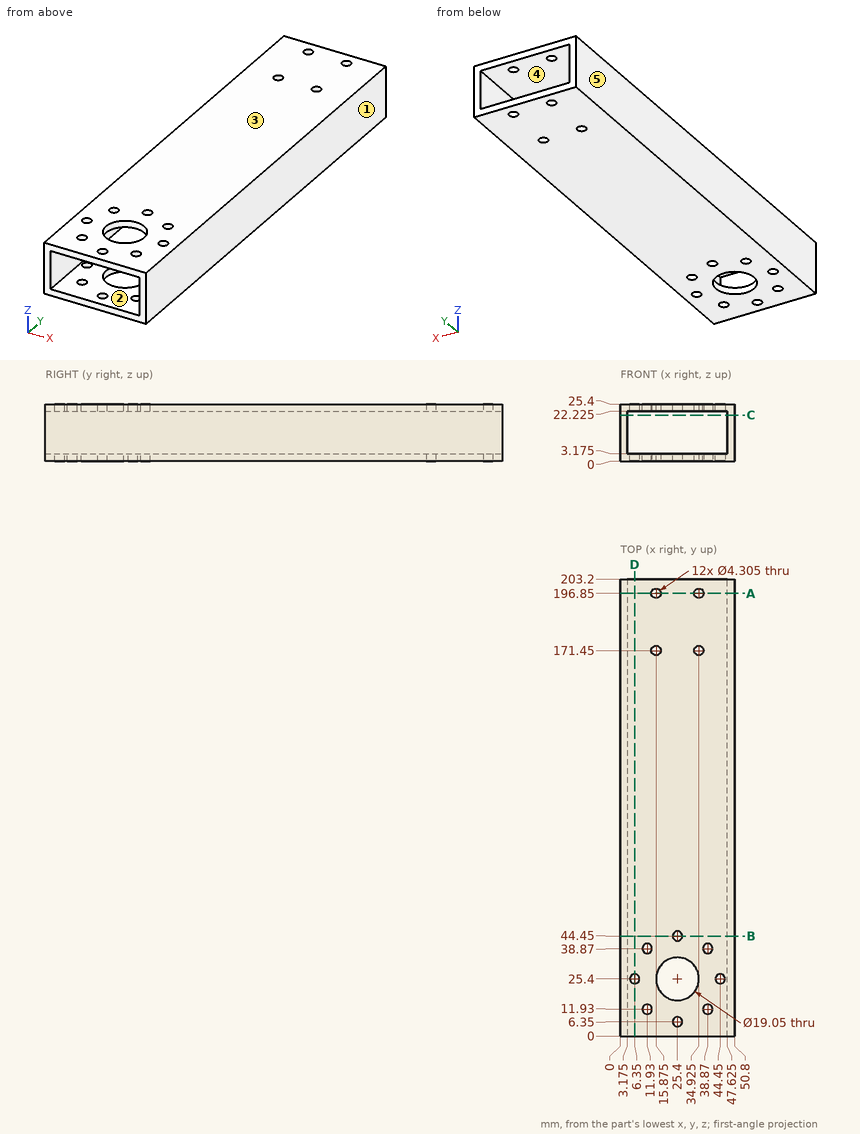
Print and shaded views of the part. All mm, measured from the part's lowest x, y and z. A direction names the side the tool comes from. Coordinates: 2 decimals unless noted, no trailing zeros. Order: outer loops, then holes, each group sorted by start corner. A loop starts at its lowest first (then second) coordinate and runs counter-clockwise, first axis right, second up. Notation, with made-up numbers: (3.5, 31) -> (23.5, 31) arc R14 cw to (23.5, 43) -> close; hole circle Ø8 at (-37.75, -13). An arc over 180 degrees is marked (long way). Answer as a JSON object with one key per item and string values. Group by question number.
1) Flat gauge pins, fed straight in: pin 1 (2.5 mm diameter, centred on x = 11.93, y = 38.87, fed in from +Z); pin 2 (7 mm diameter, centred on x = 15.875, y = 196.85, fed in from -Z). Where does each tip first touch, or does it go through?
2) Cut at C-C, the plane z = 20.5. Write the cut outline in (x, y) (1 decimal).
3) Cut at A-A, the plane y = 196.85. Write the cut outline in (x, z) (1 decimal), then the cut area to 3 significant figures.
4) Cut at B-B, the plane y = 44.45. Write the cut outline in (x, z) (1 decimal), then the cut area to 3 significant figures.
5) Drill centre lines: L1, parallel to Y at x = 25.4, z = 1.6 (1 decimal); L2, parallel to X at y = 185, z = 6.5 (1 decimal); L3, parallel to Z at x = 38, y = 27.5 (1 decimal). Where is each one in solid material? Low to high.
6) Cut at D-D, the plane x = 6.35. Write the cut outline in (y, z) (1 decimal).
7) Which spindle directions (+Z, -Z, +X, -X, +Y, -Y) get a long thin tool onto all of the face, cutting with end or side? Do the marked faces 1 and 2. Say none if no direction does.
8) Pull direction X, two halves, no side cores. Call the marked faces 3, 4 and 5: +X half, -X half, draft (parallel to the pull), parting line (faces both ways), or undercut.
Check values:
{
 "1": {"pin 1": "passes through", "pin 2": "stops at z = 0"},
 "2": {"outline": "(0, 0) -> (3.2, 0) -> (3.2, 203.2) -> (0, 203.2) -> close; (47.6, 0) -> (50.8, 0) -> (50.8, 203.2) -> (47.6, 203.2) -> close"},
 "3": {"outline": "(0, 0) -> (13.7, 0) -> (13.7, 3.2) -> (3.2, 3.2) -> (3.2, 22.2) -> (13.7, 22.2) -> (13.7, 25.4) -> (0, 25.4) -> close; (18, 0) -> (32.8, 0) -> (32.8, 3.2) -> (18, 3.2) -> close; (18, 22.2) -> (32.8, 22.2) -> (32.8, 25.4) -> (18, 25.4) -> close; (37.1, 0) -> (50.8, 0) -> (50.8, 25.4) -> (37.1, 25.4) -> (37.1, 22.2) -> (47.6, 22.2) -> (47.6, 3.2) -> (37.1, 3.2) -> close", "area": "389 mm²"},
 "4": {"outline": "(0, 0) -> (23.2, 0) -> (23.2, 3.2) -> (3.2, 3.2) -> (3.2, 22.2) -> (23.2, 22.2) -> (23.2, 25.4) -> (0, 25.4) -> close; (27.6, 0) -> (50.8, 0) -> (50.8, 25.4) -> (27.6, 25.4) -> (27.6, 22.2) -> (47.6, 22.2) -> (47.6, 3.2) -> (27.6, 3.2) -> close", "area": "416 mm²"},
 "5": {"L1": "y = 0 to 4.2, 8.5 to 15.9, 34.9 to 42.3, 46.6 to 203.2", "L2": "x = 0 to 3.2, 47.6 to 50.8", "L3": "z = 0 to 3.2, 22.2 to 25.4"},
 "6": {"outline": "(0, 0) -> (23.2, 0) -> (23.2, 3.2) -> (0, 3.2) -> close; (0, 22.2) -> (23.2, 22.2) -> (23.2, 25.4) -> (0, 25.4) -> close; (27.6, 0) -> (203.2, 0) -> (203.2, 3.2) -> (27.6, 3.2) -> close; (27.6, 22.2) -> (203.2, 22.2) -> (203.2, 25.4) -> (27.6, 25.4) -> close"},
 "7": {"face 1": "+Z, -Z, +X, +Y, -Y", "face 2": "+Y, -Y"},
 "8": {"face 3": "draft", "face 4": "undercut", "face 5": "-X half"}
}
